```python
from build123d import *

# Parameters (mm, degrees)
SKETCH1_W           = 140
SKETCH1_H           = 160
BOSS_EXTRUDE1_DEPTH = 3
SKETCH2_R           = 2
SKETCH2_R_2         = 3
CUT_EXTRUDE1_DEPTH  = 4
FILLET1_R           = 5


with BuildPart() as part:
    # Sketch1 → Boss-Extrude1 (new body)
    with BuildSketch(Plane(origin=(0, 0, 0), x_dir=(1, 0, 0), z_dir=(0, 1, 0))):
        Rectangle(SKETCH1_W, SKETCH1_H)
    extrude(amount=BOSS_EXTRUDE1_DEPTH)

    # Sketch2 → Cut-Extrude1 (cut, through all)
    with BuildSketch(Plane(origin=(0, 3, 0), x_dir=(1, 0, 0), z_dir=(0, 1, 0))):
        with Locations((-30, 26.3)):
            Circle(SKETCH2_R)
        with Locations((-30, 67.3)):
            Circle(SKETCH2_R)
        with Locations((7.5, 62.8)):
            Circle(SKETCH2_R)
        with Locations((7.5, 30.8)):
            Circle(SKETCH2_R)
        with Locations((30, -68.8)):
            Circle(SKETCH2_R)
        with Locations((-7.5, -64.3)):
            Circle(SKETCH2_R)
        with Locations((30, -27.8)):
            Circle(SKETCH2_R)
        with Locations((-7.5, -32.3)):
            Circle(SKETCH2_R)
        with Locations((46.5, -27.8)):
            Circle(SKETCH2_R)
        with Locations((46.5, -68.8)):
            Circle(SKETCH2_R)
        with Locations((-46.5, 26.3)):
            Circle(SKETCH2_R)
        with Locations((-46.5, 67.3)):
            Circle(SKETCH2_R)
        with Locations((46.5, 7.2)):
            Circle(SKETCH2_R)
        with Locations((-46.5, -8.7)):
            Circle(SKETCH2_R)
        with Locations((9.5, -65.8)):
            Circle(SKETCH2_R_2)
        with Locations((9.5, -30.8)):
            Circle(SKETCH2_R_2)
        with Locations((-9.5, 64.3)):
            Circle(SKETCH2_R_2)
        with Locations((-9.5, 29.3)):
            Circle(SKETCH2_R_2)
    extrude(amount=-CUT_EXTRUDE1_DEPTH, mode=Mode.SUBTRACT)

    # Fillet1
    fillet1_edges = [part.edges().sort_by_distance(p)[0] for p in [
        (-70, 1.5, -80),
        (70, 1.5, -80),
        (70, 1.5, 80),
        (-70, 1.5, 80),
    ]]
    fillet(fillet1_edges, radius=FILLET1_R)


solid = part.part
```
Could you check a few things on this model? Use its own coordinates, in mm. Round coordinates to 2 decimals unless told otherwise and drop trailing zeros. Write each loop counter-clockwise with the first axis right and the second up, starting at its lowest first coordinate (ties: lowest second). Pieces come first, ordered by that corner, then holes.
(1) Thinking about a two-plate mould opening in Z: for faces 1 (the face through (44.502, 1.521, -7.288)), 2 (the face through (68, 2, -79)), 3 (the face through (-8.974, 1.521, 30.948)), 4 (the face through (-69, 2, 78)), which applies, +Z half, -Z half, draft (parallel to the pull), parting line (faces both ways), or undercut?
Findings below:
face 1: undercut
face 2: -Z half
face 3: undercut
face 4: +Z half
(2) If I drill on probe 1 along Z at (x, y) = (46.5, 2.1); probe 2 along Z at (x, y) = (-12, 2.8); probe 3 along X at (y, z) = (2.2, -66.5), over which ranges is the centre line in solid material (lowest first)?
Findings below:
probe 1: z = -80 to -9.2, -5.2 to 25.8, 29.8 to 66.8, 70.8 to 80
probe 2: z = -80 to -65.96, -62.64 to -30.96, -27.64 to 80
probe 3: x = -70 to -48.33, -44.67 to -31.83, -28.17 to -11.54, -7.46 to 70
(3) Suppose I cut it at B-B on z = -7.2. Write out the boundary of the cut face in (x, y).
Findings below:
outline: (-70, 0) - (44.5, 0) - (44.5, 3) - (-70, 3) - close; (48.5, 0) - (70, 0) - (70, 3) - (48.5, 3) - close
(4) Suppose I cut it at A-A on x = 30. Write out the boundary of the cut face in (y, z).
Findings below:
outline: (0, -80) - (3, -80) - (3, 25.8) - (0, 25.8) - close; (0, 29.8) - (3, 29.8) - (3, 66.8) - (0, 66.8) - close; (0, 70.8) - (3, 70.8) - (3, 80) - (0, 80) - close
